The listing builds one solid part. Answer for the finished solid, in the listing's coordinates (mm). A direction names the side the tool comes from. Give positions to 0.01 mm unless a question says otherwise; leave off trailing zeros. Write each loop counter-clockwise with the first axis right and the second up, starting at its lowest first coordinate (ties: lowest second). Pieces come first, ordered by that corner, then holes. Notation, with made-up numbers: (-36, 4.5) - (-6, 4.5) arc R20 ccw to (-6, 21.5) - close; hole circle Ø7 at (-20.75, 14). An arc over 180 degrees is marked (long way). One line per question, with ' | ' between items. Start each with the question number.
1. A cutting plane is placed at C-C (y = 11.25). Determine the outline of the cut face in (x, z).
2. Find the intervals of material crossed by L1, parallel to Z at x = -6, y = 21.5; L2, parallel to X at y = 27, z = -15; L3, parallel to X at y = 24.75, z = -2.5, in increasing order. Write a range as from..to.
3. A cutting plane is placed at B-B (z = -2.5). Determine the outline of the cut face in (x, y), then the cut area to 3 significant figures.
4. A cutting plane is placed at A-A (y = 21.5). Determine the outline of the cut face in (x, z), then the cut area to 3 significant figures.
5. The mould has two halves that part along Z. Classify faces 3 (the face through (-7.651, 12.78, -19.912)), 4 (the face through (0, 7.85, 0)): +Z half, -Z half, draft (parallel to the pull), parting line (faces both ways), or undercut.
6. A cutting plane is placed at D-D (z = -29). Determine the outline of the cut face in (x, y).
7. Given P1, Ø3, axis at x = -12, z = 14.5, coming from the +Y side; P2, Ø2, axis at x = -12.61, z = 15.03, coming from the +Y side; P3, Ø8, axis at x = -7, z = -16, coming from the +Y side; P4, Ø5, axis at x = 6, y = 19.5, coming from the -Z side, each flat-ended and moving along its own axis, determine where each tip first touches the part or whether it passes through.
8. For faces 1 (the face through (-13.42, 12.78, -13.48)), 2 (the face through (19.393, 22.835, 6.656)), determine the directions among +Z, -Z, +X, -X, +Y, -Y from which every point of the face is accessible in a straight line to the end or side of a thin tool.
Autodesk Inventor part; units mm, degrees
ref_plane "YZ Plane" through (0, 0, 0) normal (1, 0, 0) x (0, 1, 0)
ref_plane "XZ Plane" through (0, 0, 0) normal (0, 1, 0) x (-1, 0, 0)
ref_plane "XY Plane" through (0, 0, 0) normal (0, 0, 1) x (1, 0, 0)
sketch "Szkic1" plane through (0, 0, 0) normal (0, 1, 0) x (-1, 0, 0)
  circle A0 centre (0, 0) radius 19.62 construction
  line L0 (0, 0) -> (-19.62, 0) construction
  circle A1 centre (0, 0) radius 22.5 construction
  circle A2 centre (-19.3219, 3.407) radius 1.75
  circle A3 centre (-19.3219, -3.407) radius 1.75
  circle A4 centre (6.7104, 18.4368) radius 1.75
  circle A5 centre (12.6115, 15.0298) radius 1.75
  circle A6 centre (12.6115, -15.0298) radius 1.75
  circle A7 centre (6.7104, -18.4368) radius 1.75
  circle A8 centre (0, 0) radius 35
  circle A9 centre (-19.3219, 3.407) radius 3.25
  circle A10 centre (-19.3219, -3.407) radius 3.25
  circle A11 centre (6.7104, -18.4368) radius 3.25
  circle A12 centre (12.6115, -15.0298) radius 3.25
  circle A13 centre (12.6115, 15.0298) radius 3.25
  circle A14 centre (6.7104, 18.4368) radius 3.25
  line L1 (14.2365, 17.8444) -> (8.3354, 21.2514)
  line L2 (10.9865, 12.2152) -> (5.0854, 15.6222)
  line L3 (-16.0719, 3.407) -> (-16.0719, -3.407)
  line L4 (14.2365, -17.8444) -> (8.3354, -21.2514)
  line L5 (10.9865, -12.2152) -> (5.0854, -15.6222)
  line L6 (-22.5719, -3.407) -> (-22.5719, 3.407)
  dimension "d0" = 39.24
  dimension "d1" = 3.5
  dimension "d2" = 20
  dimension "d5" = 360
  dimension "d7" = 45
  dimension "d8" = 70
  dimension "d12" = 6.5
  dimension "d15" = 360
sketch "Szkic3" plane through (0, 0, 0) normal (0, 0, 1) x (1, 0, 0)
  arc A0 (0, 35) -> (-35, 0) centre (0, 0) ccw
  line L0 (0, 35) -> (0, 0)
  line L1 (0, 0) -> (-35, 0)
  line L2 (0, -8.4497) -> (0, 50.6985)
  dimension "d19" = 35
revolve "Obrót1" add sketch "Szkic3" angle 360 about axis through (0, -10, 0) along (0, 1, 0)
extrude "Wyciągnięcie proste1" cut sketch "Szkic1" along normal through all contours A2 | A3 | A4 | A5 | A6 | A7 | A9 | L3 A10 L6 A9 | A10 | A11 | A11 L5 A12 L4 | A12 | A13 | A13 L2 A14 L1 | A14
extrude "Wyciągnięcie proste2" add sketch "Szkic1" along normal blind 17.85 contours A9 | L3 A10 L6 A9 | A10 | A11 | A11 L5 A12 L4 | A12 | A13 | A13 L2 A14 L1 | A14
extrude "Wyciągnięcie proste3" cut sketch "Szkic1" along normal blind 7.85 contours A2 | A3 | A4 | A5 | A6 | A7 | A8 | A9 | L3 A10 L6 A9 | A10 | A11 | A11 L5 A12 L4 | A12 | A13 | A13 L2 A14 L1 | A14
ref_plane "Płaszczyzna konstrukcyjna2" through (-11.286, 17.85, -19.5479) normal (-0.866, 0, 0.5) x (0.5, 0, 0.866)
properties part number "hemisphere_1"
Determined:
1) outline: circle Ø66.29 at (0, 0); hole circle Ø3.5 at (-12.61, -15.03); hole circle Ø3.5 at (-12.61, 15.03); hole circle Ø3.5 at (-6.71, -18.44); hole circle Ø3.5 at (-6.71, 18.44); hole circle Ø3.5 at (19.32, -3.41); hole circle Ø3.5 at (19.32, 3.41)
2) L1: -26.96..-21.61, -15.09..15.09, 21.61..26.96 | L2: -16.46..-15.86, -6.16..16.46 | L3: -24.62..16.07, 22.57..24.62
3) outline: (-34.02, 7.85) - (17.83, 7.85) - (17.83, 17.85) - (16.07, 17.85) - (16.07, 30.99) arc R34.91 ccw to start; (20.82, 7.85) - (34.02, 7.85) arc R34.91 ccw to (22.57, 26.63) - (22.57, 17.85) - (20.82, 17.85) - close | area: 1,270 mm2
4) outline: circle Ø55.24 at (0, 0); hole (-14.24, -17.84) - (-8.34, -21.25) arc R3.25 ccw to (-5.09, -15.62) - (-10.99, -12.22) arc R3.25 ccw to start; hole (-14.24, 17.84) arc R3.25 ccw to (-10.99, 12.22) - (-5.09, 15.62) arc R3.25 ccw to (-8.34, 21.25) - close; hole (16.07, -3.41) arc R3.25 ccw to (22.57, -3.41) - (22.57, 3.41) arc R3.25 ccw to (16.07, 3.41) - close | area: 2,160 mm2
5) face 3: undercut | face 4: draft
6) outline: (-17.95, 7.85) - (17.95, 7.85) arc R19.6 ccw to start
7) P1: y = 17.85 | P2: through | P3: y = 32.31 | P4: z = -30.08
8) face 1: +Y, -Y | face 2: +Y
